from build123d import *

# Parameters (mm, degrees)
EXTRUDE_1_DEPTH     = 13
SKETCH_3_R          = 4.25
CUT_EXTRUDE_1_DEPTH = 55.717456081
SKETCH_4_R          = 4.25
CUT_EXTRUDE_2_DEPTH = 55.717456081


with BuildPart() as part:
    # 草图1 → 凸台-拉伸1 (new, symmetric)
    with BuildSketch(Plane.XY):
        Polygon((0, 0), (40, 0), (40, 40), (37.5, 40), (35, 30), (35, 24.364950833), (35.6, 23.764950833), (35, 23.164950833), (35, 21.364950833), (35.6, 20.764950833), (35, 20.164950833), (35, 13), (27, 5), (19.835049167, 5), (19.235049167, 4.4), (18.635049167, 5), (16.835049167, 5), (16.235049167, 4.4), (15.635049167, 5), (10, 5), (0, 2.5), align=None)
    extrude(amount=EXTRUDE_1_DEPTH, both=True)

    # 草图3 → 切除-拉伸1 (cut, through all)
    with BuildSketch(Plane(origin=(0, 5, 0), x_dir=(1, 0, 0), z_dir=(0, 1, 0))):
        with Locations(Location((20, 0, 0), (0, 0, 270))):
            Circle(SKETCH_3_R)
    extrude(amount=-CUT_EXTRUDE_1_DEPTH, mode=Mode.SUBTRACT)

    # 草图4 → 切除-拉伸2 (cut, through all)
    with BuildSketch(Plane.ZY.offset(-35)):
        with Locations(Location((0, 20, 0), (0, 0, 270))):
            Circle(SKETCH_4_R)
    extrude(amount=-CUT_EXTRUDE_2_DEPTH, mode=Mode.SUBTRACT)


solid = part.part
Source: CAD feature listing. Evaluate the final solid. Frame: model axes, mm. A direction names the side the tool comes from. Give positions to 0.01 mm unless a question says otherwise; leave off trailing zeros. Loops run counter-clockwise (first coordinate to the right, second up) from the corner with the lowest first, then second, coordinate; pieces in that order, holes last. Notation, with made-up numbers: (88, -27) -> (143, -27) arc R19 cw to (143, 10) -> close; hole circle Ø10 at (64.25, 84.25). An arc over 180 degrees is marked (long way). Use a Markdown table: item, result. Add a question column.
1) Section query D-D, the plane z = 4.75. Return the cut outline in (x, y).
2) Section query A-A, the plane z = 0. Return the cut outline in (x, y), then the cut area to 3 significant figures.
3) Section query C-C, the plane x = 20.5. Return the cut outline in (y, z).
4) Line query: line 1 along Z through (x, y) = (20, 2.25); line 2 along Y through (x, z) = (38.75, 0). Output: solid intervals per line, ascending. Write a range as [from, to].
5) Section query B-B, the plane x = 37. Return the cut outline in (y, z), then the cut area to 3 significant figures.
6) Reachability of faces 4 (the face through (15, 0, 0)), 5 (the face through (35, 22, -8)) from +Z, -Z, +X, -X, +Y, -Y: full face, straight path, thin tool, end or side. Return the list, or none.
7) Pull-direction query (Z, two-part tool) for faces 1 (the face through (22.872, 2.535, -3.132)), 2 (the face through (35, 22, 8)), 3 (the face through (32, 8, 13)); classes: +Z half, -Z half, draft (parallel to the pull), parting line (faces both ways), or undercut.
8) First-contact query: pin 1 (0.9 mm diameter, centred on y = 22, z = 8.5, fed in from -X); pin 2 (3.5 mm diameter, centred on x = 24, z = 1.5, fed in from +Y); pin 3 (5 mm diameter, centred on x = 20, z = 0, fed in from +Y); pin 4 (10 mm diameter, centred on y = 12.5, z = 3.5, fed in from -X). Flat tips, straight axial feed; report the tip coordinate or a pass-through.
Numbers:
| question | item | result |
|---|---|---|
| 1 | outline | (0, 0) -> (40, 0) -> (40, 40) -> (37.5, 40) -> (35, 30) -> (35, 24.36) -> (35.6, 23.76) -> (35, 23.16) -> (35, 21.36) -> (35.6, 20.76) -> (35, 20.16) -> (35, 13) -> (27, 5) -> (19.84, 5) -> (19.24, 4.4) -> (18.64, 5) -> (16.84, 5) -> (16.24, 4.4) -> (15.64, 5) -> (10, 5) -> (0, 2.5) -> close |
| 2 | outline | (0, 0) -> (15.75, 0) -> (15.75, 4.89) -> (15.64, 5) -> (10, 5) -> (0, 2.5) -> close; (24.25, 0) -> (40, 0) -> (40, 15.75) -> (35, 15.75) -> (35, 13) -> (27, 5) -> (24.25, 5) -> close; (35, 24.36) -> (35.11, 24.25) -> (40, 24.25) -> (40, 40) -> (37.5, 40) -> (35, 30) -> close |
| 2 | area | 297 mm2 |
| 3 | outline | (0, -13) -> (5, -13) -> (5, -4.22) -> (0, -4.22) -> close; (0, 4.22) -> (5, 4.22) -> (5, 13) -> (0, 13) -> close |
| 4 | line 1 | z = [-13, -4.25], [4.25, 13] |
| 4 | line 2 | y = [0, 15.75], [24.25, 40] |
| 5 | outline | (0, -13) -> (38, -13) -> (38, 13) -> (0, 13) -> close; hole circle Ø8.5 at (20, 0) |
| 5 | area | 931 mm2 |
| 6 | face 4 | +Z, -Z, +X, -X, -Y |
| 6 | face 5 | +Z, -Z, -X, +Y |
| 7 | face 1 | undercut |
| 7 | face 2 | draft |
| 7 | face 3 | +Z half |
| 8 | pin 1 | stops at x = 35 |
| 8 | pin 2 | stops at y = 5 |
| 8 | pin 3 | passes through |
| 8 | pin 4 | stops at x = 29.5 |
